```python
from build123d import *

# Parameters (mm, degrees)
SKETCH1_R                       = 21
BOSS_EXTRUDE1_DEPTH             = 48
SKETCH2_R                       = 2.5
BOSS_EXTRUDE2_DEPTH             = 22
M3X0_5_TAPPED_HOLE1_D           = 2.5
M3X0_5_TAPPED_HOLE1_DEPTH       = 7.5
M3X0_5_TAPPED_HOLE1_CSINK_D     = 3.05
M3X0_5_TAPPED_HOLE1_CSINK_ANGLE = 90
M3X0_5_TAPPED_HOLE1_TIP         = 0.751075774
M3X0_5_TAPPED_HOLE2_D           = 2.5
M3X0_5_TAPPED_HOLE2_DEPTH       = 7.5
M3X0_5_TAPPED_HOLE2_CSINK_D     = 3.05
M3X0_5_TAPPED_HOLE2_CSINK_ANGLE = 90
M3X0_5_TAPPED_HOLE2_TIP         = 0.751075774
CHAMFER2_SIZE                   = 8.5
CHAMFER2_SIZE2                  = 4
CUT_EXTRUDE1_START              = -5
CUT_EXTRUDE1_DEPTH              = 5
SKETCH10_R                      = 5.5
BOSS_EXTRUDE3_DEPTH             = 2
CHAMFER1_SIZE                   = 1
CHAMFER3_SIZE                   = 2
SKETCH11_R                      = 17.5
CUT_EXTRUDE2_DEPTH              = 10
SKETCH12_R                      = 2
BOSS_EXTRUDE6_DEPTH             = 45
SKETCH13_R                      = 6.5
BOSS_EXTRUDE7_DEPTH             = 1


# Read off the part's stored shape, not the designer's step: Cut-Extrude1
with BuildPart() as part:
    # Sketch1 → Boss-Extrude1 (new body)
    with BuildSketch(Plane.XY):
        Circle(SKETCH1_R)
    extrude(amount=-BOSS_EXTRUDE1_DEPTH)

    # Sketch2 → Boss-Extrude2 (add)
    with BuildSketch(Plane.XY):
        Circle(SKETCH2_R)
    extrude(amount=BOSS_EXTRUDE2_DEPTH)

    # M3x0.5 Tapped Hole1
    with Locations(Plane.XY):
        with Locations((-8.838834765, -8.838834765), (-8.838834765, 8.838834765), (8.838834765, 8.838834765), (8.838834765, -8.838834765)):
            CounterSinkHole(M3X0_5_TAPPED_HOLE1_D / 2, M3X0_5_TAPPED_HOLE1_CSINK_D / 2, depth=M3X0_5_TAPPED_HOLE1_DEPTH, counter_sink_angle=M3X0_5_TAPPED_HOLE1_CSINK_ANGLE)
            with Locations((0, 0, -(M3X0_5_TAPPED_HOLE1_DEPTH + M3X0_5_TAPPED_HOLE1_TIP / 2))):  # 118° drill point
                Cone(0, M3X0_5_TAPPED_HOLE1_D / 2, M3X0_5_TAPPED_HOLE1_TIP, mode=Mode.SUBTRACT)

    # M3x0.5 Tapped Hole2
    with Locations(Plane(origin=(0, 0, -48), x_dir=(-1, 0, 0), z_dir=(0, 0, -1))):
        with Locations((0, 7.505553499), (6.5, -3.75277675), (-6.5, -3.75277675)):
            CounterSinkHole(M3X0_5_TAPPED_HOLE2_D / 2, M3X0_5_TAPPED_HOLE2_CSINK_D / 2, depth=M3X0_5_TAPPED_HOLE2_DEPTH, counter_sink_angle=M3X0_5_TAPPED_HOLE2_CSINK_ANGLE)
            with Locations((0, 0, -(M3X0_5_TAPPED_HOLE2_DEPTH + M3X0_5_TAPPED_HOLE2_TIP / 2))):  # 118° drill point
                Cone(0, M3X0_5_TAPPED_HOLE2_D / 2, M3X0_5_TAPPED_HOLE2_TIP, mode=Mode.SUBTRACT)

    # Chamfer2
    chamfer2_edges = [part.edges().sort_by_distance(p)[0] for p in [
        (-21, 0, -48),
    ]]
    chamfer2_side = [part.faces().sort_by_distance(p)[0] for p in [
        (0, 0, -48),
    ]]
    chamfer(chamfer2_edges, length=CHAMFER2_SIZE, length2=CHAMFER2_SIZE2, reference=chamfer2_side[0])

    # Cut-Extrude1 outline → Cut-Extrude1 (cut)
    with BuildSketch(Plane(origin=(0, 0, -48), x_dir=(-1, 0, 0), z_dir=(0, 0, -1)).offset(CUT_EXTRUDE1_START)):
        with BuildLine():
            ThreePointArc((20.058520203, -6.217376237), (18.1865335, 10.499999964), (4.644854416, 20.479876158))
            ThreePointArc((4.644854416, 20.479876158), (5.264488359, 13.915625351), (7.303117447, 7.645272385))
            ThreePointArc((7.303117447, 7.645272385), (7.361215932, 4.25), (10.272558828, 2.502049044))
            ThreePointArc((10.272558828, 2.502049044), (14.683529392, -2.398632152), (20.058520203, -6.217376237))
        make_face()
        with BuildLine():
            ThreePointArc((-7.303117447, 7.645272385), (-5.264488359, 13.915625351), (-4.644854416, 20.479876158))
            ThreePointArc((-4.644854416, 20.479876158), (-18.18653348, 10.5), (-20.058520227, -6.217376158))
            ThreePointArc((-20.058520227, -6.217376158), (-14.683529243, -2.398632019), (-10.272558828, 2.502049044))
            ThreePointArc((-10.272558828, 2.502049044), (-7.361215932, 4.25), (-7.303117447, 7.645272385))
        make_face()
        with BuildLine():
            ThreePointArc((-15.413665812, -14.2625), (0, -21), (15.413665812, -14.2625))
            ThreePointArc((15.413665812, -14.2625), (9.419040884, -11.516993332), (2.96944138, -10.147321429))
            ThreePointArc((2.96944138, -10.147321429), (0, -8.5), (-2.96944138, -10.147321429))
            ThreePointArc((-2.96944138, -10.147321429), (-9.419040884, -11.516993332), (-15.413665812, -14.2625))
        make_face()
    extrude(amount=CUT_EXTRUDE1_DEPTH, mode=Mode.SUBTRACT)

    # Sketch10 → Boss-Extrude3 (add)
    with BuildSketch(Plane(origin=(0, 0, -48), x_dir=(-1, 0, 0), z_dir=(0, 0, -1))):
        with Locations(Location((0, 0, 0), (0, 0, 180))):
            Circle(SKETCH10_R)
    extrude(amount=BOSS_EXTRUDE3_DEPTH)

    # Chamfer1
    chamfer1_edges = [part.edges().sort_by_distance(p)[0] for p in [
        (-5.5, 0, -50),
    ]]
    chamfer(chamfer1_edges, length=CHAMFER1_SIZE)

    # Chamfer3
    chamfer3_edges = [part.edges().sort_by_distance(p)[0] for p in [
        (-21, 0, 0),
    ]]
    chamfer(chamfer3_edges, length=CHAMFER3_SIZE)

    # Sketch11 → Cut-Extrude2 (cut)
    with BuildSketch(Plane.XY):
        with Locations((-30, 0)):
            Circle(SKETCH11_R)
        with Locations((0, 30)):
            Circle(SKETCH11_R)
        with Locations((30, 0)):
            Circle(SKETCH11_R)
    extrude(amount=-CUT_EXTRUDE2_DEPTH, mode=Mode.SUBTRACT)

    # Sketch12 → Boss-Extrude6 (add)
    with BuildSketch(Plane(origin=(0, 0, 0), x_dir=(1, 0, 0), z_dir=(0, 1, 0))):
        with Locations(Location((0, 5, 0), (0, 0, 270))):
            Circle(SKETCH12_R)
        with Locations(Location((-4.1, 5, 0), (0, 0, 270))):
            Circle(SKETCH12_R)
        with Locations(Location((4.1, 5, 0), (0, 0, 270))):
            Circle(SKETCH12_R)
    extrude(amount=-BOSS_EXTRUDE6_DEPTH)

    # Sketch13 → Boss-Extrude7 (add)
    with BuildSketch(Plane.XY):
        Circle(SKETCH13_R)
    extrude(amount=BOSS_EXTRUDE7_DEPTH)


solid = part.part
```
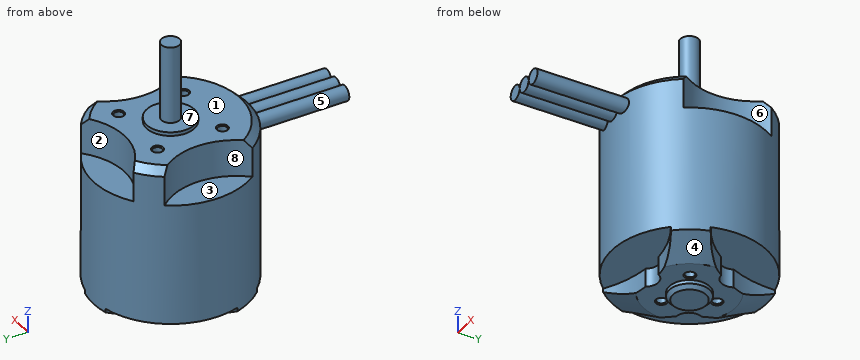
The model under review builds one solid part; all positions refer to its coordinate system, in mm. Face numbers are marked on the shaded views. A direction names the side the tool comes from. Give positions to 0.01 mm unless a question says otherwise; leave off trailing zeros. Write each loop counter-clockwise with the first axis right and the second up, starting at its lowest first coordinate (ties: lowest second). Pieces come first, ordered by that corner, then holes. Notation, with made-up numbers: M -34,21.25 L 11,21.25 A15 cw 11,37.25 Z; hole C 44.5,5.25 d8. An arc over 180 degrees is marked long. Write each question's results on one line, items separated by ' | '. Start each with the question number.
1. Insertion check: pin 1 Ø2.5 at (x, y) = (-16.5, 4) entering from +Z; pin 2 Ø3 at (x, y) = (-8.5, -29) entering from +Z; pin 3 Ø12 at (x, z) = (-16, -39.5) entering from +Y; pin 4 Ø2 at (x, y) = (-6.5, -3.75) entering from -Z. Each pin has a flat end and moves straight along its axis. Give the tip position at first contact, or say it passes through.
2. For probe 1 along X at (y, z) = (-25.5, -6); probe 2 along Z at (x, y) = (-6.5, 13.5); probe 3 along Y at (x, z) = (-12, -3.5), list the stretches that pass through material, from the lowest coordinate up. Write a range as [from, to].
3. We need section A-A (z = 4). Write out the cut boundary in (x, y).
4. For the marked faces 5, 6, 7 and 8, list the 3-axis set-ups (+Z, -Z, +X, -X, +Y, -Y) from which the entire face can be reached by the end or side of a thin tool; tool diameter is ignored.
5. We need section B-B (z = -5). Write out the cut boundary in (x, y).
6. Mouldability with a two-part tool opening along Y and no side actions: class the marked faces 1, 2, 3 and 4 as released by +Y, released by -Y, zero draft, split by the parting line, or undercut.
7. We need section C-C (z = -12.5). Write out the cut boundary in (x, y).
Results found:
1) pin 1: stops at z = -10 | pin 2: passes through | pin 3: stops at y = 18.47 | pin 4: stops at z = -40.35
2) probe 1: x = [-5.83, -2.37], [-1.73, 1.73], [2.37, 5.83] | probe 2: z = [-43, 0] | probe 3: y = [-17.23, 17.23]
3) outline: C 0,0 d5
4) face 5: -Y | face 6: +Z, +X | face 7: +Z | face 8: +Z, -X
5) outline: M -17.25,-11.98 A21 ccw -6.1,-20.09 L -6.1,-45 L -2.1,-45 L -2.1,-20.89 A21 ccw -2,-20.9 L -2,-45 L 2,-45 L 2,-20.9 A21 ccw 2.1,-20.89 L 2.1,-45 L 6.1,-45 L 6.1,-20.09 A21 ccw 17.25,-11.98 A17.5 cw 17.25,11.98 A21 ccw 11.98,17.25 A17.5 cw -11.98,17.25 A21 ccw -17.25,11.98 A17.5 cw Z; hole C -8.84,-8.84 d2.5; hole C -8.84,8.84 d2.5; hole C 8.84,-8.84 d2.5; hole C 8.84,8.84 d2.5
6) face 1: zero draft | face 2: released by +Y | face 3: undercut | face 4: released by -Y
7) outline: C 0,0 d42
